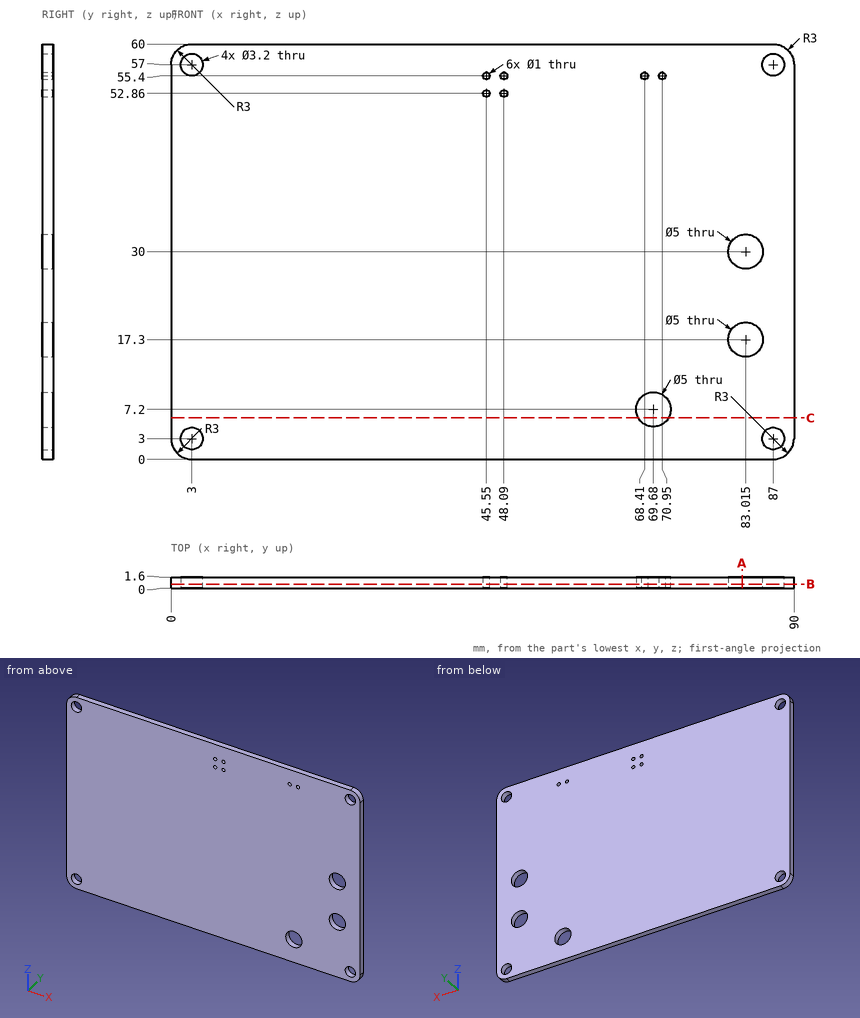
The figure shows three views and two pictorial views of one solid part (mm, origin at its lowest corner). Answer the questions. Round coordinates to 2 decimals unless told otherwise and drop trailing zeros. Write each loop counter-clockwise with the first axis right and the second up, starting at its lowest first coordinate (ties: lowest second). Pieces come first, ordered by that corner, then holes. Notation, with made-up numbers: (10, -3) - (66, -3) arc R19 ccw to (66, 4) - close; hole circle Ø6 at (70.5, 69). An arc over 180 degrees is marked (long way). Use one line per item in the form item = value. Start each with the question number.
Item 1: Find the intervals of material crossed by line 1 (X direction, y = 0.55, z = 52.86); line 2 (Z direction, x = 45.55, y = 0.4); line 3 (Z direction, x = 70.95, y = 0.55), in increasing order. Write a range as [from, to].
Item 2: A cutting plane is placed at A-A (x = 82.5). Write down the section's boundary in (y, z), plus the area to 3 significant figures.
Item 3: A cutting plane is placed at B-B (y = 0.6). Give the number of separate pieces and of enclosed holes in the cut face, plus the area to 3 significant figures.
Item 4: Flat-ended cylindrical pins translate along their axes: pin 1 Ø3.5 at (x, z) = (87, 3) entering from +Y; pin 2 Ø1.9 at (x, z) = (3, 57) entering from -Y. Find the tip coordinate at first contact, or state that the pin passes through.
Item 5: A cutting plane is placed at C-C (z = 6). Write down the section's boundary in (x, y).
The answers:
q1.line_1 = [0, 45.05], [46.05, 47.59], [48.59, 90]
q1.line_2 = [0, 52.36], [53.36, 54.9], [55.9, 60]
q1.line_3 = [0, 5.05], [9.35, 54.9], [55.9, 60]
q2.outline = (0, 0) - (1.6, 0) - (1.6, 14.85) - (0, 14.85) - close; (0, 19.75) - (1.6, 19.75) - (1.6, 27.55) - (0, 27.55) - close; (0, 32.45) - (1.6, 32.45) - (1.6, 60) - (0, 60) - close
q2.area = 80.3 mm^2
q3.separate_pieces = 1
q3.enclosed_holes = 13
q3.area = 5,300 mm^2
q4.pin_1 = 1.6
q4.pin_2 = through
q5.outline = (0, 0) - (67.49, 0) - (67.49, 1.6) - (0, 1.6) - close; (71.87, 0) - (90, 0) - (90, 1.6) - (71.87, 1.6) - close
